```python
from build123d import *

# Parameters (mm, degrees)
ESQUISSE1_R             = 175
ESQUISSE1_W             = 90
ESQUISSE1_H             = 90
BOSS_EXTRU_1_DEPTH      = 5
ENL_V_START             = -10
ENL_V_MAT_EXTRU_1_DEPTH = 10
ENL_V_MAT_EXTRU_4_DEPTH = 10


with BuildPart() as part:
    # Esquisse1 → Boss.-Extru.1 (new body)
    with BuildSketch(Plane.XY):
        Circle(ESQUISSE1_R)
        Rectangle(ESQUISSE1_W, ESQUISSE1_H, mode=Mode.SUBTRACT)
    extrude(amount=BOSS_EXTRU_1_DEPTH)

    # Esquisse2 → Enlèv. mat.-Extru.1 (cut)
    with BuildSketch(Plane.XY.offset(5).offset(ENL_V_START)):
        with BuildLine():
            Line((-156.468184794, 78.375424383), (-90, 40))
            Line((-90, 40), (-90, -40))
            Line((-90, -40), (-156.468184794, -78.375424383))
            ThreePointArc((-156.468184794, -78.375424383), (-175, 0), (-156.468184794, 78.375424383))
        make_face()
    extrude(amount=ENL_V_MAT_EXTRU_1_DEPTH, mode=Mode.SUBTRACT)

    # Esquisse3 → Enlèv. mat.-Extru.4 (cut)
    with BuildSketch(Plane.XY.offset(5).offset(ENL_V_START)):
        with BuildLine():
            Line((-156.468184794, 78.375424383), (-95.196152423, 43))
            Line((-95.196152423, 43), (-200, 43))
            Line((-200, 43), (-200, -207))
            Line((-200, -207), (200, -207))
            Line((200, -207), (200, 43))
            Line((200, 43), (169.634902069, 43))
            ThreePointArc((169.634902069, 43), (18.873149539, 173.979321261), (-156.468184794, 78.375424383))
        make_face()
        with BuildLine():
            Line((-55.235857919, 43), (55.235857919, 43))
            ThreePointArc((55.235857919, 43), (0, 70), (-55.235857919, 43))
        make_face(mode=Mode.SUBTRACT)
    extrude(amount=ENL_V_MAT_EXTRU_4_DEPTH, mode=Mode.SUBTRACT)


solid = part.part
```
For this review, take the finished solid that the model builds, in its own axes (mm). A direction names the side the tool comes from. Coordinates: 2 decimals unless noted, no trailing zeros. Loops run counter-clockwise (first coordinate to the right, second up) from the corner with the lowest first, then second, coordinate; pieces in that order, holes last.
1. Add section C-C, the plane x = 11. Give the boundary of the cut face in (y, z), then the cut area to 3 significant figures.
2. Mouldability with a two-part tool opening along X and no side actions: class faces 3 (the flat face through (-50, 43, 2)), 4 (the flat face through (-1, 45, 2)), 5 (the cylindrical face through (0.891, 69.994, 2.465)) as +X half, -X half, draft (parallel to the pull), parting line (faces both ways), or undercut.
3. Add section A-A, the plane z = 0.8. Give the boundary of the cut face in (x, y).
4. For faces 1 (the flat face through (-45, 44, 2)), 2 (the flat face through (50, 43, 2)), list the 3-axis set-ups (+Z, -Z, +X, -X, +Y, -Y) from which the entire face can be reached by the end or side of a thin tool; tool diameter is ignored.
5. For line 1 (Y direction, x = 7, z = 3.2); line 2 (X direction, y = 52.75, z = 1); line 3 (Y direction, x = 16, z = 4.15), list the stretches that pass through material, from the lowest coordinate up.
6. Add section B-B, the plane y = 49. Give the boundary of the cut face in (x, z), then the cut area to 3 significant figures.
7. Insertion check: P1, Ø3, axis at y = 46, z = 2, coming from the -X side; P2, Ø3, axis at y = 63.5, z = 3, coming from the -X side; P3, Ø1, axis at y = 54.5, z = 3, coming from the -X side. Each pin has a flat end and moves straight along its axis. Give the tip position at first contact, or say it passes through.
Result:
1. outline: (45, 0) - (69.13, 0) - (69.13, 5) - (45, 5) - close
1. area: 121 mm2
2. face 3: draft
2. face 4: undercut
2. face 5: parting line
3. outline: (-55.24, 43) - (-45, 43) - (-45, 45) - (45, 45) - (45, 43) - (55.24, 43) arc R70 ccw to start
4. face 1: +Z, -Z, -Y
4. face 2: +Z, -Z, +X, -X, -Y
5. line 1: y = 45 to 69.65
5. line 2: x = -46.02 to 46.02
5. line 3: y = 45 to 68.15
6. outline: (-49.99, 0) - (49.99, 0) - (49.99, 5) - (-49.99, 5) - close
6. area: 500 mm2
7. P1: stops at x = -54.03
7. P2: stops at x = -32.5
7. P3: stops at x = -44.54
